Source: CAD feature listing. Evaluate the final solid. Frame: model axes, mm. Round coordinates to 2 decimals unless told otherwise and drop trailing zeros. Loops run counter-clockwise (first coordinate to the right, second up) from the corner with the lowest first, then second, coordinate; pieces in that order, holes last. Notation, with made-up numbers: M 55.5,-17.5 L 78.5,-17.5 A18 ccw 78.5,1.5 Z; hole C 40,60 d3. An arc over 180 degrees is marked long. Answer as a JSON object with one key per item and string values.
from build123d import *

# Parameters (mm, degrees)
SKETCH1_R           = 14.2875
BOSS_EXTRUDE4_DEPTH = 6.35
FILLET3_R           = 25.4


with BuildPart() as part:
    # Sketch1 → Boss-Extrude4 (new body)
    with BuildSketch(Plane(origin=(0, 0, 0), x_dir=(1, 0, 0), z_dir=(0, 1, 0))):
        Polygon((-125.816166367, -9.912218002), (4.759892389, 59.225159329), (4.759892389, 211.625159329), (-131.188630818, 269.487781998), (-300.040107611, 269.487781998), (-300.040107611, -9.912218002), align=None)
        with Locations((-249.240107611, 244.087781998)):
            Circle(SKETCH1_R, mode=Mode.SUBTRACT)
        with Locations((-249.240107611, 15.487781998)):
            Circle(SKETCH1_R, mode=Mode.SUBTRACT)
    extrude(amount=BOSS_EXTRUDE4_DEPTH)

    # Fillet3
    fillet3_edges = [part.edges().sort_by_distance(p)[0] for p in [
        (-300.040107611, 3.175, 9.912218002),
        (-300.040107611, 3.175, -269.487781998),
        (-131.188630818, 3.175, -269.487781998),
        (4.759892389, 3.175, -211.625159329),
        (4.759892389, 3.175, -59.225159329),
        (-125.816166367, 3.175, 9.912218002),
    ]]
    fillet(fillet3_edges, radius=FILLET3_R)


solid = part.part
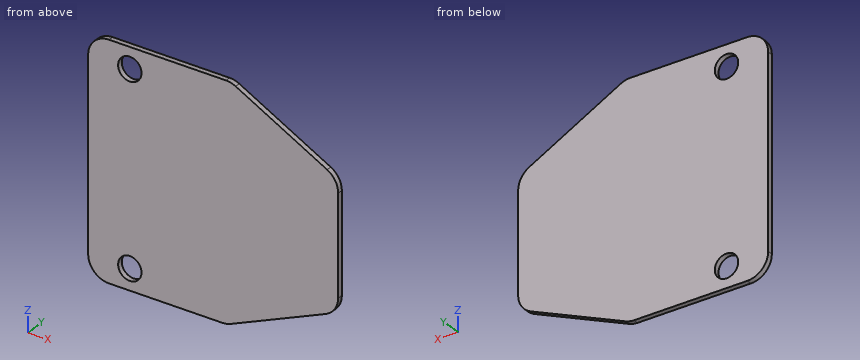
Item 1: Section D-D on z = -214.5. Return the cut outline in (x, y), then the cut area to 3 significant figures.
Answer sheet:
{"outline": "M -300.04,0 L -4.57,0 L -4.57,6.35 L -300.04,6.35 Z", "area": "1,880 mm²"}
Item 2: Section B-B on z = -8. Return the cut outline in (x, y), then the cut area to 3 significant figures.
Answer sheet:
{"outline": "M -298.91,0 L -261.41,0 L -261.41,6.35 L -298.91,6.35 Z; M -237.07,0 L -91.99,0 L -91.99,6.35 L -237.07,6.35 Z", "area": "1,160 mm²"}
Item 3: Line query: probe 1 along Z at (x, y) = (-249, 1.25); probe 2 along Z at (x, y) = (-245, 3.25); probe 3 along Z at (x, y) = (-276.5, 2.5). Output: solid intervals per line, ascending. Write a range as from..to.
Answer sheet:
{"probe 1": "z = -269.49..-258.37, -229.8..-29.77, -1.2..9.91", "probe 2": "z = -269.49..-257.73, -230.44..-29.13, -1.84..9.91", "probe 3": "z = -269.42..9.84"}
Item 4: Section C-C on x = -19. Return the cut outline in (y, z), then the cut area to 3 significant figures.
Answer sheet:
{"outline": "M 0,-221.74 L 6.35,-221.74 L 6.35,-46.64 L 0,-46.64 Z", "area": "1,110 mm²"}
Item 5: Contact query for a flat-ended pin moving along its axis: pin 1 Ø1.5 at (x, y) = (-105.5, 4) entering from -Z. Output: stop coordinate, or through.
Answer sheet:
{"pin 1": "stops at z = -258.87"}
Item 6: Section A-A on y = 2.5. Return the cut outline in (x, z) (1 decimal), then the cut area to 3 significant figures.
Answer sheet:
{"outline": "M -300,-244.1 A25.4 ccw -274.6,-269.5 L -136.4,-269.5 A25.4 ccw -126.4,-267.5 L -10.7,-218.2 A25.4 ccw 4.8,-194.8 L 4.8,-74.5 A25.4 ccw -8.8,-52.1 L -120.2,7 A25.4 ccw -132.1,9.9 L -274.6,9.9 A25.4 ccw -300,-15.5 Z; hole C -249.2,-244.1 d28.6; hole C -249.2,-15.5 d28.6", "area": "75,100 mm²"}
